from build123d import *

# Parameters (mm, degrees)
BOSS_EXTRUDE1_DEPTH = 9.975


with BuildPart() as part:
    # Sketch1 → Boss-Extrude1 (new, symmetric)
    with BuildSketch(Plane.XY):
        with BuildLine():
            Line((20.217281255, -38.799092726), (20.217281255, -5.434329714))
            ThreePointArc((20.217281255, -5.434329714), (20.583178789, -3.998535787), (21.591617389, -2.912977499))
            Line((21.591617389, -2.912977499), (31.77916921, 3.655535531))
            ThreePointArc((31.77916921, 3.655535531), (32.11531541, 4.017388294), (32.237281255, 4.495986269))
            Line((32.237281255, 4.495986269), (32.237281255, 43.700907274))
            ThreePointArc((32.237281255, 43.700907274), (31.358601598, 45.822227617), (29.237281255, 46.700907274))
            Line((29.237281255, 46.700907274), (-35.802718745, 46.700907274))
            ThreePointArc((-35.802718745, 46.700907274), (-37.924039089, 45.822227617), (-38.802718745, 43.700907274))
            Line((-38.802718745, 43.700907274), (-38.802718745, 4.495986269))
            ThreePointArc((-38.802718745, 4.495986269), (-38.6807529, 4.017388294), (-38.344606701, 3.655535531))
            Line((-38.344606701, 3.655535531), (-28.157054879, -2.912977499))
            ThreePointArc((-28.157054879, -2.912977499), (-27.14861628, -3.998535787), (-26.782718745, -5.434329714))
            Line((-26.782718745, -5.434329714), (-26.782718745, -38.799092726))
            Line((-26.782718745, -38.799092726), (20.217281255, -38.799092726))
        make_face()
    extrude(amount=BOSS_EXTRUDE1_DEPTH, both=True)


solid = part.part
Input: part model. Units: mm. Frame: model coordinates. A direction names the side the tool comes from. Coordinates: 2 decimals unless noted, no trailing zeros. Order: outer loops, then holes, each group sorted by start corner. A loop starts at its lowest first (then second) coordinate and runs counter-clockwise, first axis right, second up.
1. Access query for faces 1 (the flat face through (-4, 5, -9.975)), 2 (the flat face through (-26.783, -22, 0)), 3 (the flat face through (20.217, -22, 0)). Directions: +Z, -Z, +X, -X, +Y, -Y. A direction counts if a zero-diameter tool reaches every point of the face in a straight line with its end or side. Return the directions, or none.
Checked values:
face 1: -Z, +X, -X, +Y, -Y
face 2: +Z, -Z, -X, -Y
face 3: +Z, -Z, +X, -Y
2. Cut plane A-A, the plane z = -0.5. Return loops of the section in (x, y), plus the area to 3 significant figures.
Checked values:
outline: (-38.8, 4.5) arc R1 ccw to (-38.34, 3.66) - (-28.16, -2.91) arc R3 cw to (-26.78, -5.43) - (-26.78, -38.8) - (20.22, -38.8) - (20.22, -5.43) arc R3 cw to (21.59, -2.91) - (31.78, 3.66) arc R1 ccw to (32.24, 4.5) - (32.24, 43.7) arc R3 ccw to (29.24, 46.7) - (-35.8, 46.7) arc R3 ccw to (-38.8, 43.7) - close
area: 5,140 mm2
3. Draft query along Y for faces 4 (the flat face through (-3, 46.701, 0)), 5 (the cylindrical face through (20.57, -4.02, 0.14)), 6 (the flat face through (32.237, 24, 0)). Return one class per face: +Y half, -Y half, draft (parallel to the pull), parting line (faces both ways), or undercut.
Checked values:
face 4: +Y half
face 5: -Y half
face 6: draft
4. Cut plane B-B, the plane y = -7.5. Return loops of the section in (x, z) (3 decimals).
Checked values:
outline: (-26.783, -9.975) - (20.217, -9.975) - (20.217, 9.975) - (-26.783, 9.975) - close
5. Contact query for flat-ended pins moving along their axis: P1, Ø6, axis at x = -30.5, z = 2, coming from the -Y side; P2, Ø2, axis at y = -29, z = -6.5, coming from the +X side; P3, Ø4, axis at y = 1.5, z = 4.5, coming from the -X side. Output: stop coordinate, or through.
Checked values:
P1: stops at y = -3.49
P2: stops at x = 20.22
P3: stops at x = -38.1
6. Ray query, line 1 along X through (y, z) = (-32, -3.75); line 2 along Y through (x, z) = (22, 1.5); line 3 along Y through (x, z) = (21, 1.5). Return the intervals inside material, ascending.
Checked values:
line 1: x = -26.78 to 20.22
line 2: y = -2.65 to 46.7
line 3: y = -3.41 to 46.7
